The listing builds one solid part. Answer for the finished solid, in the listing's coordinates (mm). A direction names the side the tool comes from. Coordinates: 2 decimals unless noted, no trailing zeros. Loops run counter-clockwise (first coordinate to the right, second up) from the corner with the lowest first, then second, coordinate; pieces in that order, holes last. Notation, with made-up numbers: (7.25, -37) - (42.25, -37) arc R23 cw to (42.25, -14) - close; hole circle Ø4 at (-33.5, 74). An arc over 180 degrees is marked (long way). One line per question, with ' | ' between items.
Autodesk Inventor part; units mm, degrees
ref_plane "YZ Plane" through (0, 0, 0) normal (1, 0, 0) x (0, 1, 0)
ref_plane "XZ Plane" through (0, 0, 0) normal (0, 1, 0) x (-1, 0, 0)
ref_plane "XY Plane" through (0, 0, 0) normal (0, 0, 1) x (1, 0, 0)
sketch "Skizze1" plane through (0, 0, 0) normal (0, 1, 0) x (-1, 0, 0)
  line L0 (0, 0) -> (0, 8)
  line L1 (0, 8) -> (2, 8)
  line L2 (2, 8) -> (2, 4)
  line L3 (2, 4) -> (39, 4)
  line L4 (39, 4) -> (39, 0)
  line L5 (0, 0) -> (13.2064, 0)
  line L6 (0, 0) -> (0, -8)
  line L7 (0, -8) -> (2, -8)
  line L8 (2, -8) -> (2, -4)
  line L9 (2, -4) -> (39, -4)
  line L10 (39, -4) -> (39, 0)
  dimension "d1" = 8
  dimension "d2" = 2
  dimension "d3" = 4
  dimension "d4" = 37
extrude "Extrusion1" add sketch "Skizze1" along normal mid plane 100
sketch "Skizze5" plane through (-39, -50, 4) normal (0, 0, 1) x (1, 0, 0)
  line L0 (0, 0) -> (0, 100)
  line L1 (0, 0) -> (3.5, 0)
  line L2 (3.5, 0) -> (3.5, 20)
  line L3 (3.5, 20) -> (0, 20)
  line L4 (0, 20) -> (0, 0)
  point P0 (39, 50)
  point P1 (0, 20.0912)
  dimension "d22" = 3.5
  dimension "d23" = 20
extrude "Extrusion3" add sketch "Skizze5" along normal blind 20 and the other way blind 30
sketch "Skizze6" plane through (-39, 50, 4) normal (0, 0, 1) x (1, 0, 0)
  line L0 (0, -80) -> (0, 0)
  line L1 (0, 0) -> (3.5, 0)
  line L2 (3.5, 0) -> (3.5, -20)
  line L3 (3.5, -20) -> (0, -20)
  line L4 (0, -20) -> (0, 0)
  point P0 (39, -50)
  point P1 (0, -19.9088)
  point P2 (0, -20)
  dimension "d26" = 20
  dimension "d32" = 3.5
extrude "Extrusion4" add sketch "Skizze6" along normal blind 20 and the other way blind 30
sketch "Esquisse11" plane through (-35.5, 30, -4) normal (1, 0, 0) x (0, 0, -1)
  line L0 (22, 20) -> (0, 20)
  line L1 (22, 20) -> (22, 0)
  line L2 (22, -60) -> (22, -80)
  point P0 (-4, -30)
  point P1 (13, 7)
  point P2 (13, -67)
  dimension "d57" = 13
  dimension "d58" = 74
  dimension "d59" = 9
  dimension "d60" = 9
hole "Perçage3" at (-35.5, 37, -17) at (-35.5, -37, -17) direction (-1, 0, 0) diameter 4.917 end through all
sketch "Esquisse21" plane through (-35.5, -50, 4) normal (1, 0, 0) x (0, 0, -1)
  line L0 (0, 100) -> (0, 80)
  line L1 (0, 20) -> (0, 80)
  line L2 (0, 20) -> (0, 0)
  line L3 (0, 100) -> (0, 0)
  line L4 (-36.3372, 0) -> (0, 0)
  line L5 (0, 0) -> (0, 115.7943)
  line L6 (0, 115.7943) -> (-36.3372, 115.7943)
  line L7 (-36.3372, 115.7943) -> (-36.3372, 0)
  point P0 (4, 50)
  point P1 (0, 20)
extrude "Extrusion15" cut sketch "Esquisse21" along normal mid plane 9999
sketch "Esquisse28" plane through (0, 50, 0) normal (0, 1, 0) x (1, 0, 0)
  line L0 (-2, 4) -> (-35.5, 4)
  line L1 (-4.0336, 4) -> (2.9868, 4)
  line L2 (2.9868, 4) -> (2.9868, 11.523)
  line L3 (2.9868, 11.523) -> (-4.0336, 11.523)
  line L4 (-4.0336, 11.523) -> (-4.0336, 4)
  point P0 (0, 0)
extrude "Extrusion20" cut sketch "Esquisse28" against normal through all
sketch "Esquisse29" plane through (-35.5, -50, -4) normal (1, 0, 0) x (0, 0, -1)
  circle A0 centre (13, 87) radius 2.4585
  line L0 (0, 80) -> (0, 100)
  line L1 (0, 80) -> (22, 80)
  line L2 (22, 100) -> (22, 80)
  line L3 (22, 100) -> (0, 100)
  circle A1 centre (13, 13) radius 2.4585 construction
  line L4 (0, 0) -> (0, 20) construction
  line L5 (22, 0) -> (0, 0) construction
  line L6 (22, 20) -> (22, 0) construction
  line L7 (0, 20) -> (22, 20) construction
  point P0 (-4, 50)
extrude "Extrusion21" add sketch "Esquisse29" along normal up to surface (35.5 mm away)
sketch "Esquisse30" plane through (0, -50, -4) normal (0, 0, -1) x (-1, 0, 0)
  line L0 (39, 80) -> (0, 80)
  line L1 (35.5, 0) -> (0, 0)
  line L2 (0, 80) -> (10, 80)
  line L3 (10, 80) -> (10, 0)
  line L4 (10, 0) -> (0, 0)
  line L5 (0, 0) -> (0, 80)
  point P0 (0, 0)
  dimension "d128" = 10
extrude "Extrusion22" add sketch "Esquisse30" along normal up to surface (22 mm away)
sketch "Esquisse31" plane through (-35.5, -30, -4) normal (0, 0, -1) x (-1, 0, 0)
  line L0 (8.9947, 60) -> (-25.5, 60)
  line L1 (-25.5, 60) -> (-25.5, -26.2912)
  line L2 (-25.5, -26.2912) -> (8.9947, -26.2912)
  line L3 (8.9947, -26.2912) -> (8.9947, 60)
  point P0 (-35.5, 30)
extrude "Extrusion23" cut sketch "Esquisse31" along normal blind 100 and the other way blind 100
sketch "Esquisse32" plane through (-39, 50, -26) normal (0, 0, -1) x (-1, 0, 0)
  line L0 (-24.4847, -70) -> (-46.2931, -70)
  line L1 (-46.2931, -70) -> (-46.2931, -103.0341)
  line L2 (-46.2931, -103.0341) -> (-24.4847, -103.0341)
  line L3 (-24.4847, -103.0341) -> (-24.4847, -70)
  line L4 (-29, -100) -> (-39, -100)
  point P0 (-39, -50)
  dimension "d137" = 30
extrude "Extrusion24" cut sketch "Esquisse32" against normal through all
sketch "Esquisse33" plane through (0, 50, 0) normal (0, 1, 0) x (1, 0, 0)
  line L0 (0, -4) -> (0, 26)
  line L1 (-39, 26) -> (-39, -4)
  line L2 (0, -4) -> (-39, -4)
  line L3 (-39, -4) -> (-39, 11)
  line L4 (-39, 11) -> (0, 11)
  line L5 (0, 11) -> (0, -4)
  point P0 (0, 0)
  point P1 (-39, -4)
extrude "Extrusion25" cut sketch "Esquisse33" against normal through all
sketch "Esquisse34" plane through (-10, -20, -26) normal (-1, 0, 0) x (0, 0, 1)
  line L0 (7.7873, 42) -> (7.7873, 12) construction
  line L1 (5.2873, 42) -> (5.2873, 12)
  line L2 (10.2873, 12) -> (10.2873, 42)
  arc A0 (10.2873, 42) -> (5.2873, 42) centre (7.7873, 42) ccw
  arc A1 (5.2873, 12) -> (10.2873, 12) centre (7.7873, 12) ccw
  line L3 (0, 0) -> (15, 0)
  line L4 (0, 50) -> (15, 50)
  point P0 (26, 20)
  point P1 (7.7873, 27)
  dimension "d141" = 8
  dimension "d142" = 5
  dimension "d151" = 30
extrude "Extrusion26" cut sketch "Esquisse34" against normal through all
sketch "Esquisse35" plane through (0, 50, 0) normal (0, 1, 0) x (1, 0, 0)
  line L0 (-1, 5.3347) -> (8.2352, 5.3347)
  line L1 (8.2352, 5.3347) -> (8.2352, 39.622)
  line L2 (8.2352, 39.622) -> (-1, 39.622)
  line L3 (-1, 39.622) -> (-1, 5.3347)
  line L4 (0, 11) -> (0, 26)
  point P0 (0, 0)
  dimension "d145" = 1
extrude "Extrusion27" cut sketch "Esquisse35" against normal through all
sketch "Esquisse36" plane through (-39, 50, -26) normal (0, 0, -1) x (-1, 0, 0)
  line L0 (7.4978, 8.0322) -> (-50.8948, 8.0322)
  line L1 (-50.8948, 8.0322) -> (-50.8948, -8)
  line L2 (-50.8948, -8) -> (7.4978, -8)
  line L3 (7.4978, -8) -> (7.4978, 8.0322)
  line L4 (0, 0) -> (-38, 0)
  point P0 (-39, -50)
  dimension "d148" = 8
extrude "Extrusion28" cut sketch "Esquisse36" against normal through all
sketch "Esquisse37" plane through (-39, 50, -26) normal (0, 0, -1) x (-1, 0, 0)
  line L0 (-23.4802, -64) -> (-55.2745, -64)
  line L1 (-55.2745, -64) -> (-55.2745, -79.7659)
  line L2 (-55.2745, -79.7659) -> (-23.4802, -79.7659)
  line L3 (-23.4802, -79.7659) -> (-23.4802, -64)
  line L4 (-38, -70) -> (-29, -70)
  point P0 (-39, -50)
  dimension "d152" = 6
extrude "Extrusion29" cut sketch "Esquisse37" against normal through all
properties part number "Befestigung Bremssattel"
Item 1: Find section D-D, the plane y = -0.5. Write down the section's boundary in (x, z).
Taken from the geometry:
outline: (-10, -26) - (-1, -26) - (-1, -20.71) - (-10, -20.71) - close; (-10, -15.71) - (-1, -15.71) - (-1, -11) - (-10, -11) - close
Item 2: The mould has two halves that part along Y. Classify faces 1 (the face through (-6, 7, -15.713)), 2 (the face through (-8, 27, -11)), 3 (the face through (-25, 30, -18)), 4 (the face through (-5.6, -10.5, -18.3)): pulls with the +Y half, pulls with the -Y half, needs draft (parallel to the pull), parting line crosses it, or undercut.
Taken from the geometry:
face 1: undercut | face 2: needs draft | face 3: pulls with the -Y half | face 4: undercut
Item 3: Find the intervals of material crossed by line 1 (Y direction, x = -18, z = -17); line 2 (Y direction, x = -4.5, z = -18.75); line 3 (Z direction, x = -29.5, y = 37), in increasing order. Write a range as [from, to].
Taken from the geometry:
line 1: y = [30, 34.54], [39.46, 42] | line 2: y = [-14, -10.44], [24.44, 35.27], [38.73, 42] | line 3: z = [-26, -19.46], [-14.54, -11]
Item 4: Find section B-B, the plane z = -17. Write down the section's boundary in (x, y), plus the area to 3 significant figures.
Taken from the geometry:
outline: (-39, 30) - (-10, 30) - (-10, 24.19) - (-1, 24.19) - (-1, 34.54) - (-39, 34.54) - close; (-39, 39.46) - (-1, 39.46) - (-1, 42) - (-39, 42) - close; (-10, -14) - (-1, -14) - (-1, -10.19) - (-10, -10.19) - close | area: 356 mm2
Item 5: This flat-tipped pin is pushed along its axis until it touches: pin 1 Ø4.5 at (y, z) = (15, -21) entering from -X. Where does it stop, or does it pass through?
Taken from the geometry:
pin 1: stops at x = -10
Item 6: Find section A-A, the plane y = 37. Write down the section's boundary in (x, z).
Taken from the geometry:
outline: (-39, -26) - (-1, -26) - (-1, -19.46) - (-39, -19.46) - close; (-39, -14.54) - (-1, -14.54) - (-1, -11) - (-39, -11) - close
Item 7: Find section C-C, the plane x = -19. Write down the section's boundary in (y, z), plus the area to 3 significant figures.
Taken from the geometry:
outline: (30, -26) - (42, -26) - (42, -11) - (30, -11) - close; hole circle Ø4.92 at (37, -17) | area: 161 mm2
Item 8: Which of the six approach directions +Z, -Z, +X, -X, +Y, -Y give full straight-line access (tool end or side, diameter ignored) to faces 5 (the face through (-39, 34.6, -18.4)), 6 (the face through (-5.6, 24.5, -18.2)), 7 (the face through (-10, 8, -15))?
Taken from the geometry:
face 5: +Z, -Z, -X, +Y, -Y | face 6: +X, -X | face 7: +Z, -Z, -X, -Y
